```python
from build123d import *

# Parameters (mm, degrees)
SKETCH_1_W          = 36
SKETCH_1_H          = 60
EXTRUDE_1_DEPTH     = 18
FILLET_1_R          = 2
SHELL_START         = -16
SHELL_1_OUTLINE_W   = 16
SHELL_1_OUTLINE_H   = 56
SHELL_1_DEPTH       = 32
SKETCH_2_W          = 25
SKETCH_2_H          = 2
EXTRUDE_2_DEPTH     = 12
SKETCH_3_R          = 3
CUT_EXTRUDE_1_DEPTH = 14
SKETCH_4_R          = 3
EXTRUDE_3_DEPTH     = 18
FILLET_2_R          = 3
SKETCH_6_W          = 25
SKETCH_6_H          = 2
EXTRUDE_4_DEPTH     = 12
SKETCH_8_R          = 3
CUT_EXTRUDE_2_DEPTH = 14
SKETCH_9_R          = 1.4
CUT_EXTRUDE_3_DEPTH = 10
SKETCH_11_R         = 1.4
CUT_EXTRUDE_5_DEPTH = 66
SKETCH_13_R         = 5.125
CUT_EXTRUDE_6_DEPTH = 66
SKETCH_14_R         = 5.125
CUT_EXTRUDE_7_DEPTH = 66


# Read off the part's stored shape, not the designer's step: 抽壳1
with BuildPart() as part:
    # 草图1 → 凸台-拉伸1 (new body)
    with BuildSketch(Plane(origin=(0, 0, 0), x_dir=(1, 0, 0), z_dir=(0, 1, 0))):
        Rectangle(SKETCH_1_W, SKETCH_1_H)
    extrude(amount=EXTRUDE_1_DEPTH)

    # 圆角1
    fillet_1_edges = [part.edges().sort_by_distance(p)[0] for p in [
        (-18, 9, -30),
        (18, 9, -30),
        (18, 9, 30),
        (-18, 9, 30),
    ]]
    fillet(fillet_1_edges, radius=FILLET_1_R)

    # 抽壳1 outline → 抽壳1 (cut)
    with BuildSketch(Plane.YZ.offset(SHELL_START)):
        with Locations((10, 0)):
            Rectangle(SHELL_1_OUTLINE_W, SHELL_1_OUTLINE_H)
    extrude(amount=SHELL_1_DEPTH, mode=Mode.SUBTRACT)

    # 草图2 → 凸台-拉伸2 (add)
    with BuildSketch(Plane(origin=(0, 2, 0), x_dir=(1, 0, 0), z_dir=(0, 1, 0))):
        with Locations((3.5, -16.5)):
            Rectangle(SKETCH_2_W, SKETCH_2_H)
    extrude(amount=EXTRUDE_2_DEPTH)

    # 草图3 → 切除-拉伸1 (cut)
    with BuildSketch(Plane(origin=(18, 0, 0), x_dir=(0, 0, -1), z_dir=(1, 0, 0))):
        with Locations((-22.75, 8.5)):
            Circle(SKETCH_3_R)
    extrude(amount=-CUT_EXTRUDE_1_DEPTH, mode=Mode.SUBTRACT)

    # 草图4 → 凸台-拉伸3 (add)
    with BuildSketch(Plane(origin=(0, 18, 0), x_dir=(1, 0, 0), z_dir=(0, 1, 0))):
        with Locations((0, 32)):
            Circle(SKETCH_4_R)
        with Locations((0, -32)):
            Circle(SKETCH_4_R)
    extrude(amount=-EXTRUDE_3_DEPTH)

    # 圆角2
    fillet_2_edges = [part.edges().sort_by_distance(p)[0] for p in [
        (2.236067977, 9, -30),
        (-2.236067977, 9, -30),
        (-2.236067977, 9, 30),
        (2.236067977, 9, 30),
    ]]
    fillet(fillet_2_edges, radius=FILLET_2_R)

    # 草图6 → 凸台-拉伸4 (add)
    with BuildSketch(Plane(origin=(0, 2, 0), x_dir=(1, 0, 0), z_dir=(0, 1, 0))):
        with Locations((-3.5, 16.5)):
            Rectangle(SKETCH_6_W, SKETCH_6_H)
    extrude(amount=EXTRUDE_4_DEPTH)

    # 草图8 → 切除-拉伸2 (cut)
    with BuildSketch(Plane.ZY.offset(18)):
        with Locations((-22.75, 8.5)):
            Circle(SKETCH_8_R)
    extrude(amount=-CUT_EXTRUDE_2_DEPTH, mode=Mode.SUBTRACT)

    # 草图9 → 切除-拉伸3 (cut)
    with BuildSketch(Plane(origin=(0, 18, 0), x_dir=(1, 0, 0), z_dir=(0, 1, 0))):
        with Locations(Location((0, 32, 0), (0, 0, 270))):
            Circle(SKETCH_9_R)
        with Locations(Location((0, -32, 0), (0, 0, 270))):
            Circle(SKETCH_9_R)
    extrude(amount=-CUT_EXTRUDE_3_DEPTH, mode=Mode.SUBTRACT)

    # 草图11 → 切除-拉伸5 (cut)
    with BuildSketch(Plane(origin=(18, 0, 0), x_dir=(0, 0, -1), z_dir=(1, 0, 0))):
        with Locations((-8, 14.6)):
            Circle(SKETCH_11_R)
        with Locations((0, 14.6)):
            Circle(SKETCH_11_R)
        with Locations((8, 14.6)):
            Circle(SKETCH_11_R)
    extrude(amount=-CUT_EXTRUDE_5_DEPTH, mode=Mode.SUBTRACT)

    # 草图13 → 切除-拉伸6 (cut)
    with BuildSketch(Plane.ZY.offset(-16)):
        with Locations((-22.75, 8.5)):
            Circle(SKETCH_13_R)
    extrude(amount=-CUT_EXTRUDE_6_DEPTH, mode=Mode.SUBTRACT)

    # 草图14 → 切除-拉伸7 (cut)
    with BuildSketch(Plane(origin=(-16, 0, 0), x_dir=(0, 0, -1), z_dir=(1, 0, 0))):
        with Locations((-22.75, 8.5)):
            Circle(SKETCH_14_R)
    extrude(amount=-CUT_EXTRUDE_7_DEPTH, mode=Mode.SUBTRACT)


solid = part.part
```
The listing builds one solid part. Answer for the finished solid, in the listing's coordinates (mm). A direction names the side the tool comes from. Round coordinates to 2 decimals unless told otherwise and drop trailing zeros. Order: outer loops, then holes, each group sorted by start corner. A loop starts at its lowest first (then second) coordinate and runs counter-clockwise, first axis right, second up. Notation, with made-up numbers: (10, 66) -> (17, 66) arc R26 ccw to (17, 105) -> close; hole circle Ø10 at (11, -17). An arc over 180 degrees is marked (long way). Answer as CSV lines item,"result".
Q1. Which of the six approach directions +Z, -Z, +X, -X, +Y, -Y give full straight-line access (tool end or side, diameter ignored) to faces 1 (the cylindrical face through (16.99, 10.04, -17.86)), 2 (the flat face through (-11, 9, 30)), 3 (the cylindrical face through (0.06, 13.07, 30.6))?
Computed values:
face 1,"+X"
face 2,"+Z, -X, +Y, -Y"
face 3,"+Y"
Q2. A cutting plane is placed at B-B on x = 0. Determine the outline of the cut face in (y, z).
Computed values:
outline,"(0, -35) -> (18, -35) -> (18, -33.4) -> (8, -33.4) -> (8, -30.6) -> (18, -30.6) -> (18, -28) -> (2, -28) -> (2, -17.5) -> (14, -17.5) -> (14, -15.5) -> (2, -15.5) -> (2, 15.5) -> (14, 15.5) -> (14, 17.5) -> (2, 17.5) -> (2, 28) -> (18, 28) -> (18, 30.6) -> (8, 30.6) -> (8, 33.4) -> (18, 33.4) -> (18, 35) -> (0, 35) -> close"
Q3. Consider line 1 (Z direction, x = 8, y = 8.5); line 2 (Z direction, x = 14.5, y = 2.5); line 3 (Y direction, x = 16.9, z = 8). Determine where each line is inside the solid, lowest interval first. Write a range as from..to.
Computed values:
line 1,"z = -30..-28, -17.5..-15.5, 15.5..17.5, 28..30"
line 2,"z = -30..-28, 15.5..17.5, 28..30"
line 3,"y = 0..13.2, 16..18"
Q4. A cutting plane is placed at C-C on z = -11. Determine the outline of the cut face in (x, y).
Computed values:
outline,"(-18, 0) -> (18, 0) -> (18, 18) -> (16, 18) -> (16, 2) -> (-16, 2) -> (-16, 18) -> (-18, 18) -> close"
Q5. Given pin 1 (8 mm diameter, centred on x = -11, y = 10.5, fed in from +Z); pin 2 (10 mm diameter, centred on x = 0.5, z = -19, fed in from +Y); pin 3 (2 mm diameter, centred on x = -4, z = 14, fed in from +Y), each flat-ended and moving along its own axis, determine where each tip first touches the part or whether it passes through.
Computed values:
pin 1,"stops at z = 30"
pin 2,"stops at y = 14"
pin 3,"stops at y = 2"
Q6. A cutting plane is placed at D-D on z = 22.75. Determine the outline of the cut face in (x, y) (3 decimals), plus the area to 4 significant figures.
Computed values:
outline,"(-18, 0) -> (18, 0) -> (18, 5.5) -> (16, 5.5) -> (16, 2) -> (-16, 2) -> (-16, 3.375) -> (-18, 3.375) -> close; (-18, 13.625) -> (-16, 13.625) -> (-16, 18) -> (-18, 18) -> close; (16, 11.5) -> (18, 11.5) -> (18, 18) -> (16, 18) -> close"
area,"103.5 mm^2"
Q7. For a pull along Z with two mould halves and no side action, classify faces 4 (the flat face through (-18, 9, 0)), 5 (the flat face through (0, 10, -28)), 6 (the cylindrical face through (17.43, 9.13, -29.4)) as +Z half, -Z half, draft (parallel to the pull), parting line (faces both ways), or undercut.
Computed values:
face 4,"draft"
face 5,"undercut"
face 6,"-Z half"
Q8. A cutting plane is placed at A-A on z = 0. Determine the outline of the cut face in (x, y).
Computed values:
outline,"(-18, 0) -> (18, 0) -> (18, 13.2) -> (16, 13.2) -> (16, 2) -> (-16, 2) -> (-16, 13.2) -> (-18, 13.2) -> close; (-18, 16) -> (-16, 16) -> (-16, 18) -> (-18, 18) -> close; (16, 16) -> (18, 16) -> (18, 18) -> (16, 18) -> close"
